```python
from build123d import *

# Parameters (mm, degrees)
SKETCH_1_W          = 28
SKETCH_1_H          = 24
EXTRUDE_2_DEPTH     = 12
SKETCH_2_W          = 24
SKETCH_2_H          = 20
CUT_EXTRUDE_1_DEPTH = 7
SKETCH_3_W          = 24
SKETCH_3_H          = 3
EXTRUDE_4_DEPTH     = 6
HOLE_WIZARD_1_D     = 3.5
HOLE_WIZARD_2_D     = 2.3
SKETCH_10_W         = 2.5
SKETCH_10_H         = 7
CUT_EXTRUDE_2_DEPTH = 1
CUT_EXTRUDE_3_DEPTH = 3.2


with BuildPart() as part:
    # 草图1 → 凸台-拉伸2 (new body)
    with BuildSketch(Plane(origin=(0, 0, 0), x_dir=(1, 0, 0), z_dir=(0, 1, 0))):
        Rectangle(SKETCH_1_W, SKETCH_1_H)
    extrude(amount=EXTRUDE_2_DEPTH)

    # 草图2 → 切除-拉伸1 (cut)
    with BuildSketch(Plane(origin=(0, 12, 0), x_dir=(1, 0, 0), z_dir=(0, 1, 0))):
        Rectangle(SKETCH_2_W, SKETCH_2_H)
    extrude(amount=-CUT_EXTRUDE_1_DEPTH, mode=Mode.SUBTRACT)

    # 草图3 → 凸台-拉伸4 (add)
    with BuildSketch(Plane.ZY.offset(14)):
        with Locations((0, 1.5)):
            Rectangle(SKETCH_3_W, SKETCH_3_H)
    extrude_4 = extrude(amount=EXTRUDE_4_DEPTH)

    # 孔1 (through all)
    with Locations(Plane(origin=(0, 3, 0), x_dir=(1, 0, 0), z_dir=(0, 1, 0))):
        with Locations((-17, 9), (-17, -9)):
            hole_wizard_1 = Hole(HOLE_WIZARD_1_D / 2)

    # 镜向1: 凸台-拉伸4, 孔1 across plane
    add(extrude_4.mirror(Plane.ZY))
    add(hole_wizard_1.mirror(Plane.ZY), mode=Mode.SUBTRACT)

    # 孔2 (through all)
    with Locations(Plane(origin=(0, 5, 0), x_dir=(1, 0, 0), z_dir=(0, 1, 0))):
        with Locations((9.5, 7.5), (9.5, -7.5)):
            Hole(HOLE_WIZARD_2_D / 2)

    # 草图10 → 切除-拉伸2 (cut)
    with BuildSketch(Plane(origin=(0, 5, 0), x_dir=(1, 0, 0), z_dir=(0, 1, 0))):
        with Locations((10.75, 0)):
            Rectangle(SKETCH_10_W, SKETCH_10_H)
    extrude(amount=-CUT_EXTRUDE_2_DEPTH, mode=Mode.SUBTRACT)

    # 草图11 → 切除-拉伸3 (cut)
    with BuildSketch(Plane(origin=(0, 0, 0), x_dir=(-1, 0, 0), z_dir=(0, -1, 0))):
        Polygon((-11.924871131, -7.5), (-10.712435565, -9.6), (-8.287564435, -9.6), (-7.075128869, -7.5), (-8.287564435, -5.4), (-10.712435565, -5.4), align=None)
        Polygon((-11.924871131, 7.5), (-10.712435565, 5.4), (-8.287564435, 5.4), (-7.075128869, 7.5), (-8.287564435, 9.6), (-10.712435565, 9.6), align=None)
    extrude(amount=-CUT_EXTRUDE_3_DEPTH, mode=Mode.SUBTRACT)


solid = part.part
```
The listing builds one solid part. Answer for the finished solid, in the listing's coordinates (mm). A direction names the side the tool comes from. Give positions to 0.01 mm unless a question says otherwise; leave off trailing zeros. Loops run counter-clockwise (first coordinate to the right, second up) from the corner with the lowest first, then second, coordinate; pieces in that order, holes last. Notation, with made-up numbers: (35, -11) - (66, -11) arc R18 ccw to (66, 24) - close; hole circle Ø1 at (-40, 36). An arc over 180 degrees is marked (long way). Return JSON: item names as keys, results as strings. Group by question number.
1. Find section D-D (x = -4). Write down the section's boundary in (y, z), then the cut area to 3 significant figures.
2. Find section A-A (x = 17). Write down the section's boundary in (y, z).
3. Which of the six approach directions +Z, -Z, +X, -X, +Y, -Y give full straight-line access (tool end or side, diameter ignored) to faces 1 (the flat face through (17, 3, 0)), 2 (the flat face through (11.31, 1.578, 6.435)), 3 (the flat face through (0, 9, -10)), 4 (the flat face through (-14, 7, 0))?
4. Find section C-C (y = 11.25). Write down the section's boundary in (x, z), then the cut area to 3 significant figures.
5. Determine the mould class of faces 5 (the flat face through (14, 7, 0)), 6 (the flat face through (0, 5, 0)), 7 (the flat face through (0, 6, 12)) for opening direction Z: pulls with the +Z half, pulls with the -Z half, needs draft (parallel to the pull), parting line crosses it, or undercut.
6. Given pin 1 Ø1 at (x, z) = (-7.5, 6.5) entering from +Y; pin 2 Ø3.5 at (x, z) = (9.5, -7.5) entering from -Y; pin 3 Ø3.5 at (y, z) = (9.5, -3) entering from +X; pin 4 Ø1 at (x, z) = (9, -1) entering from -Y, each flat-ended and moving along its own axis, determine where each tip first touches the part or whether it passes through.
7. Straight lines are drawn through the part: line 1 (Z direction, x = -17, y = 2.35); line 2 (X direction, y = 5.75, z = -5.25); line 3 (Z direction, x = -7, y = 5.75). For each, find the intervals that lie inside material, in ascending order. Write a range as [from, to].
8. Find section B-B (z = 8). Write down the section's boundary in (x, y), then the cut area to 3 significant figures.
Verdict:
{
 "1": {"outline": "(0, -12) - (12, -12) - (12, -10) - (5, -10) - (5, 10) - (12, 10) - (12, 12) - (0, 12) - close", "area": "148 mm^2"},
 "2": {"outline": "(0, -12) - (3, -12) - (3, -10.75) - (0, -10.75) - close; (0, -7.25) - (3, -7.25) - (3, 7.25) - (0, 7.25) - close; (0, 10.75) - (3, 10.75) - (3, 12) - (0, 12) - close"},
 "3": {"face 1": "+Z, -Z, +X, +Y", "face 2": "-Y", "face 3": "+Y", "face 4": "+Z, -Z, -X, +Y"},
 "4": {"outline": "(-14, -12) - (14, -12) - (14, 12) - (-14, 12) - close; hole (-12, -10) - (12, -10) - (12, 10) - (-12, 10) - close", "area": "192 mm^2"},
 "5": {"face 5": "needs draft", "face 6": "undercut", "face 7": "pulls with the +Z half"},
 "6": {"pin 1": "stops at y = 5", "pin 2": "stops at y = 3.2", "pin 3": "stops at x = 14", "pin 4": "stops at y = 0"},
 "7": {"line 1": "z = [-12, -10.75], [-7.25, 7.25], [10.75, 12]", "line 2": "x = [-14, -12], [12, 14]", "line 3": "z = [-12, -10], [10, 12]"},
 "8": {"outline": "(-20, 0) - (-18.44, 0) - (-18.44, 3) - (-20, 3) - close; (-15.56, 0) - (7.36, 0) - (7.36, 3.2) - (8.46, 3.2) - (8.46, 5) - (-12, 5) - (-12, 12) - (-14, 12) - (-14, 3) - (-15.56, 3) - close; (10.54, 3.2) - (11.64, 3.2) - (11.64, 0) - (15.56, 0) - (15.56, 3) - (14, 3) - (14, 12) - (12, 12) - (12, 5) - (10.54, 5) - close; (18.44, 0) - (20, 0) - (20, 3) - (18.44, 3) - close", "area": "169 mm^2"}
}
